The listing builds one solid part. Answer for the finished solid, in the listing's coordinates (mm). Give positions to 0.01 mm unless a question says otherwise; leave off trailing zeros. Order: outer loops, then holes, each group sorted by start corner. A loop starts at its lowest first (then second) coordinate and runs counter-clockwise, first axis right, second up. Notation, with made-up numbers: M 39.25,-9.75 L 74.25,-9.75 A29 cw 74.25,25.25 Z; hole C -39,1 d2. An arc over 180 degrees is marked long. Answer as a JSON object with one key per item and string values. Group by question number.
```python
from build123d import *

# Parameters (mm, degrees)
SKETCH_1_R      = 1.25
EXTRUDE_1_DEPTH = 6
CHAMFER_1_SIZE  = 0.3


with BuildPart() as part:
    # 草图1 → 凸台-拉伸1 (new body)
    with BuildSketch(Plane.YZ):
        Polygon((2.655811238, 0), (1.327905619, 2.3), (-1.327905619, 2.3), (-2.655811238, 0), (-1.327905619, -2.3), (1.327905619, -2.3), align=None)
        with Locations(Location((0, 0, 0), (0, 0, 270))):
            Circle(SKETCH_1_R, mode=Mode.SUBTRACT)
    extrude(amount=EXTRUDE_1_DEPTH)

    # 倒角1
    chamfer_1_edges = [part.edges().sort_by_distance(p)[0] for p in [
        (6, 0, 2.3),
        (6, -1.991858429, 1.15),
        (0, 0, 1.25),
        (6, 0, 1.25),
        (6, -1.991858429, -1.15),
        (6, 0, -2.3),
        (6, 1.991858429, -1.15),
        (0, 0, -2.3),
        (0, -1.991858429, -1.15),
        (0, -1.991858429, 1.15),
        (0, 0, 2.3),
        (0, 1.991858429, 1.15),
        (0, 1.991858429, -1.15),
        (6, 1.991858429, 1.15),
    ]]
    chamfer(chamfer_1_edges, length=CHAMFER_1_SIZE)


solid = part.part
```
Item 1: Consider probe 1 along Y at (x, z) = (2.65, -0.95); probe 2 along Z at (x, y) = (2.35, -0.75); probe 3 along Y at (x, z) = (1.7, 0.4). Determine where each line is inside the solid, lowest interval first. Write a range as from..to.
Item 2: Section B-B (x = 4.5) is taken. Determine the outline of the cut face in (y, z).
Item 3: Section C-C (z = 1.65) is taken. Determine the outline of the cut face in (x, y), and give its area (3 significant figures).
Item 4: Determine the mould class of faces 1 (the flat face through (2.96, -1.98, 1.17)), 2 (the cylindrical face through (2.96, -1.22, 0.27)), 3 (the flat face through (0, 2, 0)) for opening direction Z: released by +Z, released by -Z, zero draft, split by the parting line, or undercut.
Item 5: Flat-ended cylindrical pins translate along their axes: P1, Ø2, axis at y = 0, z = -1, coming from the -X side; P2, Ø1.5, axis at y = 0, z = 0, coming from the +X side; P3, Ø2, axis at x = 1.5, z = 0.5, coming from the -Y side. Find the tip coordinate at first contact, or state that the pin passes through.
Item 6: Section A-A (y = 0) is taken. Determine the outline of the cut face in (x, z).
Values found:
{
 "1": {"probe 1": "y = -2.11..-0.81, 0.81..2.11", "probe 2": "z = -2.3..-1, 1..2.3", "probe 3": "y = -2.42..-1.18, 1.18..2.42"},
 "2": {"outline": "M -2.66,0 L -1.33,-2.3 L 1.33,-2.3 L 2.66,0 L 1.33,2.3 L -1.33,2.3 Z; hole C 0,0 d2.5"},
 "3": {"outline": "M 0,-1.36 L 0.3,-1.7 L 5.7,-1.7 L 6,-1.36 L 6,1.36 L 5.7,1.7 L 0.3,1.7 L 0,1.36 Z", "area": "20.2 mm^2"},
 "4": {"face 1": "released by +Z", "face 2": "undercut", "face 3": "zero draft"},
 "5": {"P1": "stops at x = 0", "P2": "passes through", "P3": "stops at y = -2.66"},
 "6": {"outline": "M 0,-2 L 0.3,-2.3 L 5.7,-2.3 L 6,-2 L 6,-1.55 L 5.7,-1.25 L 0.3,-1.25 L 0,-1.55 Z; M 0,1.55 L 0.3,1.25 L 5.7,1.25 L 6,1.55 L 6,2 L 5.7,2.3 L 0.3,2.3 L 0,2 Z"}
}
